```python
from build123d import *

# Parameters (mm, degrees)
SKETCH1_W           = 35
SKETCH1_H           = 35
BOSS_EXTRUDE1_DEPTH = 355
SKETCH1_3_R         = 8.057610329
BOSS_EXTRUDE2_DEPTH = 30
SKETCH1_4_R         = 8.057610329
BOSS_EXTRUDE3_DEPTH = 60
SKETCH2_W           = 20
SKETCH2_H           = 20
BOSS_EXTRUDE4_DEPTH = 20
CUT_EXTRUDE1_REACH  = 362.939
SKETCH3_R           = 4


with BuildPart() as part:
    # Sketch1 → Boss-Extrude1 (new body)
    with BuildSketch(Plane(origin=(0, 0, 0), x_dir=(1, 0, 0), z_dir=(0, 1, 0))):
        Rectangle(SKETCH1_W, SKETCH1_H)
    extrude(amount=BOSS_EXTRUDE1_DEPTH)

    # Sketch1_3 → Boss-Extrude2 (add)
    with BuildSketch(Plane(origin=(0, 0, 0), x_dir=(1, 0, 0), z_dir=(0, 1, 0))):
        with BuildLine():
            ThreePointArc((41.626297716, 17.5), (59.126297716, 0), (41.626297716, -17.5))
            Line((41.626297716, -17.5), (17.5, -17.5))
            Line((17.5, -17.5), (17.5, 17.5))
            Line((17.5, 17.5), (41.626297716, 17.5))
        make_face()
        with Locations(Location((41.626297716, 0, 0), (0, 0, 270))):
            Circle(SKETCH1_3_R, mode=Mode.SUBTRACT)
    extrude(amount=BOSS_EXTRUDE2_DEPTH)

    # Sketch1_4 → Boss-Extrude3 (add)
    with BuildSketch(Plane(origin=(0, 0, 0), x_dir=(1, 0, 0), z_dir=(0, 1, 0))):
        with Locations(Location((41.626297716, 0, 0), (0, 0, 270))):
            Circle(SKETCH1_4_R)
    extrude(amount=BOSS_EXTRUDE3_DEPTH)

    # Sketch2 → Boss-Extrude4 (add)
    with BuildSketch(Plane.XZ):
        Rectangle(SKETCH2_W, SKETCH2_H)
    extrude(amount=BOSS_EXTRUDE4_DEPTH)

    # Sketch3 → Cut-Extrude1 (cut, up to next)
    with BuildSketch(Plane.XY.offset(10), mode=Mode.PRIVATE) as cut_extrude1_sk1:
        with Locations((0, -9.583237288)):
            Circle(SKETCH3_R)
    cut_extrude1_tool1 = extrude(cut_extrude1_sk1.sketch, amount=-CUT_EXTRUDE1_REACH, mode=Mode.PRIVATE) & part.part
    add(cut_extrude1_tool1.solids().sort_by_distance((0, -9.583237, 10))[0], mode=Mode.SUBTRACT)


solid = part.part
```
Can you work these out from the model? Positions are in its coordinate system, mm. A direction names the side the tool comes from. Coordinates: 2 decimals unless noted, no trailing zeros. Order: outer loops, then holes, each group sorted by start corner. A loop starts at its lowest first (then second) coordinate and runs counter-clockwise, first axis right, second up.
1. If we section it at A-A (x = 0): Please give me the cut outline in (y, z).
2. If we section it at D-D (x = 29): Please give me the cut outline in (y, z).
3. I'm going to push flat-ended pins straight in: pin 1 (10 mm diameter, centred on y = 141, z = 0, fed in from +X); pin 2 (6 mm diameter, centred on x = 1.5, y = -6, fed in from -Z); pin 3 (17.5 mm diameter, centred on x = 45, z = 4, fed in from +Y); pin 4 (7 mm diameter, centred on x = 0, y = -9.58, fed in from -Z). Where does each tip first touch, or does it pass through?
4. I need wall thicknesses on line 1 (Y direction, x = 0, z = 5.25); line 2 (Y direction, x = 32, z = -5); line 3 (X direction, y = 172, z = -6). Which ranges of each line are inside material? Lowest first, please.
5. For faces 5 (the face through (0, -5, -10)), 6 (the face through (10, -10, 0)), 7 (the face through (0, -5, 10)), 8 (the face through (42, 60, 0)), 9 (the face through (33.76, 44.79, -1.75)), which set-ups out of +Z, -Z, +X, -X, +Y, -Y let a thin tool reach every point of the face, with its end or its side?
6. Thinking about a two-plate mould opening in Y: for faces 1 (the face through (34, 30, -4)), 2 (the face through (-0.867, -13.488, 0.14)), 3 (the face through (17.5, 190, 0)), 4 (the face through (0, -20, 0)), which applies, +Y half, -Y half, draft (parallel to the pull), parting line (faces both ways), or undercut?
7. If we section it at C-C (y = 302): Please give me the cut outline in (x, z).
8. If we section it at B-B (z = 0): Please give me the cut outline in (x, y).
Entries:
1. outline: (-20, -10) - (-13.58, -10) - (-13.58, 10) - (-20, 10) - close; (-5.58, -10) - (0, -10) - (0, -17.5) - (355, -17.5) - (355, 17.5) - (0, 17.5) - (0, 10) - (-5.58, 10) - close
2. outline: (0, -17.5) - (30, -17.5) - (30, 17.5) - (0, 17.5) - close
3. pin 1: stops at x = 17.5
3. pin 2: stops at z = -10
3. pin 3: stops at y = 60
3. pin 4: passes through
4. line 1: y = -20 to -13.58, -5.58 to 355
4. line 2: y = 0 to 30
4. line 3: x = -17.5 to 17.5
5. face 5: -Z, +X, -X, -Y
5. face 6: +Z, -Z, +X, -Y
5. face 7: +Z, +X, -X, -Y
5. face 8: +Z, -Z, +X, +Y
5. face 9: +Y
6. face 1: +Y half
6. face 2: undercut
6. face 3: draft
6. face 4: -Y half
7. outline: (-17.5, -17.5) - (17.5, -17.5) - (17.5, 17.5) - (-17.5, 17.5) - close
8. outline: (-17.5, 0) - (-10, 0) - (-10, -20) - (10, -20) - (10, 0) - (59.13, 0) - (59.13, 30) - (49.68, 30) - (49.68, 60) - (33.57, 60) - (33.57, 30) - (17.5, 30) - (17.5, 355) - (-17.5, 355) - close; hole circle Ø8 at (0, -9.58)
